```python
from build123d import *

# Parameters (mm, degrees)
F0_W      = 200
F0_H      = 300
F1_DEPTH  = 1.5
F2_W      = 20
F2_H      = 300
F3_DEPTH  = 200
F4_W      = 20
F4_H      = 300
F5_DEPTH  = 200
F6_W      = 199.424341321
F6_H      = 299.7533082962
F7_DEPTH  = 20
F9_W      = 198.1611847878
F9_H      = 219.8059260845
F10_DEPTH = 20
F11_W     = 200
F11_H     = 220
F12_DEPTH = 20
F13_R     = 38.1050822629
F14_DEPTH = 20


with BuildPart() as f1:
    # F0 (on Front) → F1 (new body)
    with BuildSketch(Plane.XZ):
        with Locations((100, 150)):
            Rectangle(F0_W, F0_H)
    extrude(amount=F1_DEPTH)

    # F2 (on Front) → F3 (join)
    with BuildSketch(Plane.XZ):
        with Locations((10, 150)):
            Rectangle(F2_W, F2_H)
    extrude(amount=F3_DEPTH)

    # F4 (on face) → F5 (join)
    with BuildSketch(Plane.XZ.offset(1.5)):
        with Locations((190, 150)):
            Rectangle(F4_W, F4_H)
    extrude(amount=F5_DEPTH)

    # F6 (on face) → F7 (join)
    with BuildSketch(Plane.XZ.offset(200)):
        with Locations((99.7121706605, 149.8766541481)):
            Rectangle(F6_W, F6_H)
    extrude(amount=F7_DEPTH)

    # F9 (on face) → F10 (join)
    with BuildSketch(Plane.XY.offset(300)):
        with Locations((99.0805923939, -109.9029630423)):
            Rectangle(F9_W, F9_H)
    extrude(amount=F10_DEPTH)

    # F11 (on face) → F12 (join)
    with BuildSketch(Plane(origin=(0, 0, 0), x_dir=(1, 0, 0), z_dir=(0, 0, -1))):
        with Locations((100, 110)):
            Rectangle(F11_W, F11_H)
    extrude(amount=F12_DEPTH)

    # F13 (on face) → F14 (cut)
    with BuildSketch(Plane.XZ.offset(220)):
        with Locations((102.2598743439, 85.0789397955)):
            Circle(F13_R)
    extrude(amount=-F14_DEPTH, mode=Mode.SUBTRACT)


solid = f1.part
```
Work out the finished part from the listing and answer in its coordinate system (mm). A direction names the side the tool comes from. Give positions to 0.01 mm unless a question says otherwise; leave off trailing zeros. Order: outer loops, then holes, each group sorted by start corner. A loop starts at its lowest first (then second) coordinate and runs counter-clockwise, first axis right, second up. Notation, with made-up numbers: (23, 37.5) - (61, 37.5) arc R26 cw to (61, 61.5) - close; hole circle Ø5 at (17.25, 86). An arc over 180 degrees is marked (long way). One line per item, written item: value. Start each with the question number.
1. Section B-B, the plane x = 51.5 is taken. Write down the section's boundary in (y, z).
2. Consider line 1 (X direction, y = -106, z = 160.5); line 2 (Y direction, x = 125.5, z = 288); line 3 (Z direction, x = 50, y = -77.5). Determine where each line is inside the solid, lowest interval first.
3. Section D-D, the plane x = 77.5 is taken. Write down the section's boundary in (y, z).
4. Each of these flat-tipped pins is pushed along its axis until it touches: pin 1 Ø10 at (x, z) = (69, 309) entering from -Y; pin 2 Ø0.5 at (x, y) = (199.5, -214) entering from +Z; pin 3 Ø22 at (y, z) = (-73.5, 311.5) entering from +X; pin 4 Ø4 at (y, z) = (-76.5, 246.5) entering from -X. Where does it stop, or does it pass through?
5. Which of the six approach directions +Z, -Z, +X, -X, +Y, -Y give full straight-line access (tool end or side, diameter ignored) to faces 1 (the face through (99, -102, 0)), 2 (the face through (94, -210.14, 47.88)), 3 (the face through (198.161, -111, 310))?
6. Section A-A, the plane y = -87 is taken. Write down the section's boundary in (x, z), then the cut area to 3 significant figures.
7. Section C-C, the plane z = 158 is taken. Write down the section's boundary in (x, y), then the cut area to 3 significant figures.
8. For a pull along X with two mould halves and no side action, classify faces 4 (the face through (199.424, -211, 148)), 5 (the face through (98, -109, 300)), 6 (the face through (0, -108, 152)), 7 (the face through (99, 0, 152)) as released by +X, released by -X, zero draft, split by the parting line, or undercut.
Filled sheet:
1. outline: (-220, -20) - (0, -20) - (0, 320) - (-219.81, 320) - (-219.81, 300) - (-1.5, 300) - (-1.5, 0) - (-200, 0) - (-200, 299.75) - (-220, 299.75) - close
2. line 1: 0 to 20, 180 to 200
2. line 2: -220 to -200, -1.5 to 0
2. line 3: -20 to 0, 300 to 320
3. outline: (-220, -20) - (0, -20) - (0, 320) - (-219.81, 320) - (-219.81, 300) - (-1.5, 300) - (-1.5, 0) - (-200, 0) - (-200, 56.11) - (-220, 56.11) - close; (-220, 114.04) - (-200, 114.04) - (-200, 299.75) - (-220, 299.75) - close
4. pin 1: y = -219.81
4. pin 2: z = 299.75
4. pin 3: x = 198.16
4. pin 4: x = 0
5. face 1: none
5. face 2: -Y
5. face 3: +Z, +X, +Y, -Y
6. outline: (0, -20) - (200, -20) - (200, 300) - (198.16, 300) - (198.16, 320) - (0, 320) - close; hole (20, 0) - (180, 0) - (180, 300) - (20, 300) - close
6. area: 20,000 mm²
7. outline: (0, -220) - (199.42, -220) - (199.42, -201.5) - (200, -201.5) - (200, 0) - (0, 0) - close; hole (20, -200) - (180, -200) - (180, -1.5) - (20, -1.5) - close
7. area: 12,200 mm²
8. face 4: released by +X
8. face 5: undercut
8. face 6: released by -X
8. face 7: zero draft
